Build history of the part. All positions in model axes, mm. A direction names the side the tool comes from. Round coordinates to 2 decimals unless told otherwise and drop trailing zeros. Loops run counter-clockwise (first coordinate to the right, second up) from the corner with the lowest first, then second, coordinate; pieces in that order, holes last. Notation, with made-up numbers: (-9, -35) - (37, -35) arc R18 ccw to (37, -5) - close; hole circle Ø2 at (38, -28). An arc over 180 degrees is marked (long way). Use one line per item in the form item = value. Start each with the question number.
Q1. Saw through at A-A (x = 13). Give the cut face in (y, z).
Q2. Saw through at B-B (y = 13.5). Give the cut face in (x, z), then the cut area to 3 significant figures.
Q3. Saw through at C-C (z = 7.5). Give the cut face in (x, y).
Q4. Mould opens along Z. For faces 1 (the face through (10, 12, 10)), 2 (the face through (23.4, 14.3, 3.2)), 3 (the face through (0, 8, 5)) say: released by +Z, released by -Z, zero draft, split by the parting line, or undercut.
Q5. Pin check, flat tips, straight feed: pin 1 (4.5 mm diameter, centred on x = 21, z = 5, fed in from -Y); pin 2 (5 mm diameter, centred on x = 21, z = 5, fed in from +Y); pin 3 (3 mm diameter, centred on x = 15.5, y = 7, fed in from -Z). Stop position of each tip, or through.
Q6. Drill centre lines: line 1 (Z direction, x = 21, y = 11.45); line 2 (Y direction, x = 13, z = 5.5); line 3 (Y direction, x = 17.5, z = 0.5). Where is each one in solid material? Low to high.
Q7. 3-axis set-ups, long thin cutter, end or side, ignore diameter. For faces 4 (the face through (23, 7, 5)), 5 (the face through (22.75, 10.77, 5.08)), 6 (the face through (19.521, 1.479, 7.608)): which of +Z, -Z, +X, -X, +Y, -Y reach the whole face in a straight line?
Q8. Saw through at D-D (x = 18.5). Give the cut face in (y, z).
```python
from build123d import *

# Parameters (mm, degrees)
PAD_DEPTH       = 10
SKETCH001_R     = 1.75
POCKET_DEPTH    = 16
SKETCH002_R     = 3
POCKET001_DEPTH = 3.5
POCKET002_DEPTH = 3


with BuildPart() as part:
    # Sketch → Pad (new body)
    with BuildSketch(Plane.XY):
        with BuildLine():
            Line((0, 0), (0, 16))
            Line((0, 16), (25, 16))
            Line((25, 16), (25, 9))
            Line((25, 9), (17.130678, 9))
            ThreePointArc((17.130678, 9), (8.75, 8), (17.130678, 7))
            Line((17.130678, 7), (25, 7))
            Line((25, 7), (25, 0))
            Line((25, 0), (0, 0))
        make_face()
    extrude(amount=PAD_DEPTH)

    # Sketch001 → Pocket (cut)
    with BuildSketch(Plane(origin=(0, 16, 0), x_dir=(-1, 0, 0), z_dir=(0, 1, 0))):
        with Locations((-21, 4.999996)):
            Circle(SKETCH001_R)
    extrude(amount=-POCKET_DEPTH, mode=Mode.SUBTRACT)

    # Sketch002 → Pocket001 (cut)
    with BuildSketch(Plane(origin=(0, 16, 0), x_dir=(-1, 0, 0), z_dir=(0, 1, 0))):
        with Locations((-21, 5)):
            Circle(SKETCH002_R)
    extrude(amount=-POCKET001_DEPTH, mode=Mode.SUBTRACT)

    # Sketch003 → Pocket002 (cut)
    with BuildSketch(Plane.XZ):
        Polygon((20.999999, 8.461405), (18, 6.729354), (18, 3.265252), (21, 1.533202), (24, 3.265253), (24, 6.729355), align=None)
    extrude(amount=-POCKET002_DEPTH, mode=Mode.SUBTRACT)


solid = part.part
```
Report:
q1.outline = (0, 0) - (3.75, 0) - (3.75, 10) - (0, 10) - close; (12.25, 0) - (16, 0) - (16, 10) - (12.25, 10) - close
q2.outline = (0, 0) - (25, 0) - (25, 10) - (0, 10) - close; hole circle Ø6 at (21, 5)
q2.area = 222 mm²
q3.outline = (0, 0) - (19.33, 0) - (19.33, 3) - (22.67, 3) - (22.67, 0) - (25, 0) - (25, 7) - (17.13, 7) arc R4.25 cw (long way) to (17.13, 9) - (25, 9) - (25, 16) - (22.66, 16) - (22.66, 12.5) - (19.34, 12.5) - (19.34, 16) - (0, 16) - close
q4.face_1 = released by +Z
q4.face_2 = undercut
q4.face_3 = zero draft
q5.pin_1 = 3
q5.pin_2 = 12.5
q5.pin_3 = through
q6.line_1 = 0 to 3.25, 6.75 to 10
q6.line_2 = 0 to 3.75, 12.25 to 16
q6.line_3 = 0 to 7, 9 to 16
q7.face_4 = +Z, -Z, +X
q7.face_5 = +Y, -Y
q7.face_6 = -Y
q8.outline = (0, 0) - (7, 0) - (7, 10) - (0, 10) - (0, 7.02) - (3, 7.02) - (3, 2.98) - (0, 2.98) - close; (9, 0) - (16, 0) - (16, 3.34) - (12.5, 3.34) - (12.5, 6.66) - (16, 6.66) - (16, 10) - (9, 10) - close
